from build123d import *

# Parameters (mm, degrees)
ESQUISSE1_W             = 40
ESQUISSE1_H             = 45
ESQUISSE1_R             = 1.75
BOSS_EXTRU_1_DEPTH      = 10
ESQUISSE2_R             = 4
ENL_V_MAT_EXTRU_2_DEPTH = 5
BOSS_EXTRU_2_DEPTH      = 10
ESQUISSE4_W             = 5
ESQUISSE4_H             = 50
BOSS_EXTRU_3_DEPTH      = 20
ENL_V_MAT_EXTRU_3_REACH = 106.163
ESQUISSE5_R             = 3.25
ESQUISSE7_R             = 2.75
BOSS_EXTRU_4_DEPTH      = 10
ENL_V_MAT_EXTRU_5_REACH = 115.719
ESQUISSE8_R             = 15
CHANFREIN1_SIZE         = 15
ENL_V_MAT_EXTRU_4_REACH = 105.475
CHANFREIN3_SIZE         = 3.5


with BuildPart() as part:
    # Esquisse1 → Boss.-Extru.1 (new body)
    with BuildSketch(Plane.XY):
        with Locations((-20, 22.5)):
            Rectangle(ESQUISSE1_W, ESQUISSE1_H)
        with Locations((-16.5, 32.5)):
            Circle(ESQUISSE1_R, mode=Mode.SUBTRACT)
        with Locations((-36.5, 32.5)):
            Circle(ESQUISSE1_R, mode=Mode.SUBTRACT)
        with Locations((-36.5, 12.5)):
            Circle(ESQUISSE1_R, mode=Mode.SUBTRACT)
        with Locations((-16.5, 12.5)):
            Circle(ESQUISSE1_R, mode=Mode.SUBTRACT)
    extrude(amount=BOSS_EXTRU_1_DEPTH)

    # Esquisse2 → Enlèv. mat.-Extru.2 (cut)
    with BuildSketch(Plane.XY.offset(10)):
        with Locations((-36.5, 32.5)):
            Circle(ESQUISSE2_R)
        with Locations((-16.5, 32.5)):
            Circle(ESQUISSE2_R)
        with Locations((-36.5, 12.5)):
            Circle(ESQUISSE2_R)
        with Locations((-16.5, 12.5)):
            Circle(ESQUISSE2_R)
    extrude(amount=-ENL_V_MAT_EXTRU_2_DEPTH, mode=Mode.SUBTRACT)

    # Esquisse3 → Boss.-Extru.2 (add)
    with BuildSketch(Plane.ZY):
        Polygon((10, 0), (45, 35), (45, 85), (40, 85), (0, 45), (10, 45), align=None)
    extrude(amount=BOSS_EXTRU_2_DEPTH)

    # Esquisse4 → Boss.-Extru.3 (add)
    with BuildSketch(Plane.ZY.offset(10)):
        with Locations((42.5, 60)):
            Rectangle(ESQUISSE4_W, ESQUISSE4_H)
    extrude(amount=BOSS_EXTRU_3_DEPTH)

    # Esquisse5 → Enlèv. mat.-Extru.3 (cut, up to next)
    with BuildSketch(Plane.XY.offset(45), mode=Mode.PRIVATE) as enl_v_mat_extru_3_sk1:
        with Locations((-21.5, 70)):
            Circle(ESQUISSE5_R)
    enl_v_mat_extru_3_tool1 = extrude(enl_v_mat_extru_3_sk1.sketch, amount=-ENL_V_MAT_EXTRU_3_REACH, mode=Mode.PRIVATE) & part.part
    # Esquisse5 → Enlèv. mat.-Extru.3 (cut, up to next)
    with BuildSketch(Plane.XY.offset(45), mode=Mode.PRIVATE) as enl_v_mat_extru_3_sk2:
        with Locations((-21.5, 50)):
            Circle(ESQUISSE5_R)
    enl_v_mat_extru_3_tool2 = extrude(enl_v_mat_extru_3_sk2.sketch, amount=-ENL_V_MAT_EXTRU_3_REACH, mode=Mode.PRIVATE) & part.part
    add(enl_v_mat_extru_3_tool1.solids().sort_by_distance((-21.5, 70, 45))[0], mode=Mode.SUBTRACT)
    add(enl_v_mat_extru_3_tool2.solids().sort_by_distance((-21.5, 50, 45))[0], mode=Mode.SUBTRACT)

    # Esquisse7 → Boss.-Extru.4 (add)
    with BuildSketch(Plane.XZ):
        Polygon((0, 0), (0, 10), (-10, 10), (-31.3834406, 29), (-43.3834406, 29), (-43.3834406, 0), align=None)
        with Locations(Location((-37.3834406, 22, 0), (0, 0, 270))):
            Circle(ESQUISSE7_R, mode=Mode.SUBTRACT)
    extrude(amount=BOSS_EXTRU_4_DEPTH)

    # Esquisse8 → Enlèv. mat.-Extru.5 (cut, up to next)
    with BuildSketch(Plane.XZ.offset(10), mode=Mode.PRIVATE) as enl_v_mat_extru_5_sk1:
        with Locations((-56.3834406, 22)):
            Circle(ESQUISSE8_R)
    enl_v_mat_extru_5_tool1 = extrude(enl_v_mat_extru_5_sk1.sketch, amount=-ENL_V_MAT_EXTRU_5_REACH, mode=Mode.PRIVATE) & part.part
    add(enl_v_mat_extru_5_tool1.solids().sort_by_distance((-56.383441, -10, 22))[0], mode=Mode.SUBTRACT)

    # Chanfrein1
    # the kernel refuses this chamfer: 15 mm, written as the material it adds along each edge
    with BuildSketch(Plane(origin=(-10, 35, 40), x_dir=(0, 0, -1), z_dir=(0, 1, 0))) as chanfrein1_piece_1_section:
        Polygon((CHANFREIN1_SIZE, 0), (0, CHANFREIN1_SIZE), (0, 0), align=None)
    chanfrein1_piece_1 = extrude(amount=88.575244819, mode=Mode.PRIVATE)
    chanfrein1_piece_1 = split(chanfrein1_piece_1, bisect_by=Plane(origin=(-10, 60, 15), z_dir=(0, -0.707106781186543, 0.7071067811865521)), keep=Keep.TOP, mode=Mode.PRIVATE)
    chanfrein1_piece_1 = chanfrein1_piece_1 - Plane(origin=(-21.5, 50, 40), x_dir=(1, 0, 0), z_dir=(0, 0, 1)) * Cylinder(3.25, 238, mode=Mode.PRIVATE)
    chanfrein1_piece_1 = chanfrein1_piece_1 - Plane(origin=(-21.5, 70, 40), x_dir=(1, 0, 0), z_dir=(0, 0, 1)) * Cylinder(3.25, 238, mode=Mode.PRIVATE)
    add(chanfrein1_piece_1)
    with BuildSketch(Plane(origin=(-10, 83.575244819, 10), x_dir=(0, 0, 1), z_dir=(0, -1, 0))) as chanfrein1_piece_2_section:
        Polygon((CHANFREIN1_SIZE, 0), (0, CHANFREIN1_SIZE), (0, 0), align=None)
    chanfrein1_piece_2 = extrude(amount=122.150489639, mode=Mode.PRIVATE)
    chanfrein1_piece_2 = split(chanfrein1_piece_2, bisect_by=Plane(origin=(-10, 69.28762241, 24.28762241), z_dir=(0, -0.707106781186543, 0.7071067811865521)), keep=Keep.TOP, mode=Mode.PRIVATE)
    chanfrein1_piece_2 = split(chanfrein1_piece_2, bisect_by=Plane(origin=(-10, 41.78762241, 51.78762241), z_dir=(0, 0.7071067811865328, -0.7071067811865622)), keep=Keep.TOP, mode=Mode.PRIVATE)
    chanfrein1_piece_2 = chanfrein1_piece_2 - Plane(origin=(-16.5, 12.5, 10), x_dir=(1, 0, 0), z_dir=(0, 0, 1)) * Cylinder(4, 305, mode=Mode.PRIVATE)
    chanfrein1_piece_2 = chanfrein1_piece_2 - Plane(origin=(-16.5, 32.5, 10), x_dir=(1, 0, 0), z_dir=(0, 0, 1)) * Cylinder(4, 305, mode=Mode.PRIVATE)
    chanfrein1_piece_2 = split(chanfrein1_piece_2, bisect_by=Plane(origin=(1.78762241, 71.78762241, 10), z_dir=(0.7071067811865477, -0.7071067811865474, 0)), keep=Keep.TOP, mode=Mode.PRIVATE)
    add(chanfrein1_piece_2)
    with BuildSketch(Plane(origin=(-10, 83.575244819, 10), x_dir=(0, 0, 1), z_dir=(0, -1, 0))) as chanfrein1_piece_3_section:
        Polygon((CHANFREIN1_SIZE, 0), (0, CHANFREIN1_SIZE), (0, 0), align=None)
    chanfrein1_piece_3 = extrude(amount=83.575244819, mode=Mode.PRIVATE)
    chanfrein1_piece_3 = split(chanfrein1_piece_3, bisect_by=Plane(origin=(-10, 41.78762241, 51.78762241), z_dir=(0, -0.7071067811865328, 0.7071067811865622)), keep=Keep.TOP, mode=Mode.PRIVATE)
    chanfrein1_piece_3 = split(chanfrein1_piece_3, bisect_by=Plane(origin=(-10, 83.575244819, 10), z_dir=(-0.6642173069108601, 0, -0.7475395435694919)), keep=Keep.TOP, mode=Mode.PRIVATE)
    add(chanfrein1_piece_3)
    with BuildSketch(Plane(origin=(-10, 45, -38.575244819), x_dir=(-1, 0, 0), z_dir=(0, 0, 1))) as chanfrein1_piece_4_section:
        Polygon((CHANFREIN1_SIZE, 0), (0, -CHANFREIN1_SIZE), (0, 0), align=None)
    chanfrein1_piece_4 = extrude(amount=87.150489639, mode=Mode.PRIVATE)
    chanfrein1_piece_4 = split(chanfrein1_piece_4, bisect_by=Plane(origin=(-10, 25.71237759, -19.28762241), z_dir=(0, -0.707106781186543, 0.7071067811865521)), keep=Keep.TOP, mode=Mode.PRIVATE)
    chanfrein1_piece_4 = split(chanfrein1_piece_4, bisect_by=Plane(origin=(-41.78762241, 45, -6.78762241), z_dir=(0.7071067811865476, 0, -0.7071067811865476)), keep=Keep.TOP, mode=Mode.PRIVATE)
    add(chanfrein1_piece_4)

    # Esquisse6 → Enlèv. mat.-Extru.4 (cut, up to next)
    with BuildSketch(Plane(origin=(0, 0, 40), x_dir=(-1, 0, 0), z_dir=(0, 0, -1)), mode=Mode.PRIVATE) as enl_v_mat_extru_4_sk1:
        with BuildLine():
            Line((13.5, 70), (13.5, 85))
            Line((13.5, 85), (29.5, 85))
            Line((29.5, 85), (29.5, 70))
            ThreePointArc((29.5, 70), (21.5, 62), (13.5, 70))
        make_face()
    enl_v_mat_extru_4_tool1 = extrude(enl_v_mat_extru_4_sk1.sketch, amount=ENL_V_MAT_EXTRU_4_REACH, mode=Mode.PRIVATE) & part.part
    # Esquisse6 → Enlèv. mat.-Extru.4 (cut, up to next)
    with BuildSketch(Plane(origin=(0, 0, 40), x_dir=(-1, 0, 0), z_dir=(0, 0, -1)), mode=Mode.PRIVATE) as enl_v_mat_extru_4_sk2:
        with BuildLine():
            Line((29.5, 50), (29.5, 35))
            Line((29.5, 35), (13.5, 35))
            Line((13.5, 35), (13.5, 50))
            ThreePointArc((13.5, 50), (21.5, 58), (29.5, 50))
        make_face()
    enl_v_mat_extru_4_tool2 = extrude(enl_v_mat_extru_4_sk2.sketch, amount=ENL_V_MAT_EXTRU_4_REACH, mode=Mode.PRIVATE) & part.part
    add(enl_v_mat_extru_4_tool1.solids().sort_by_distance((-21.5, 74.283507, 40))[0], mode=Mode.SUBTRACT)
    add(enl_v_mat_extru_4_tool2.solids().sort_by_distance((-21.5, 45.716493, 40))[0], mode=Mode.SUBTRACT)

    # Chanfrein3
    # the kernel refuses this chamfer: 3.5 mm, written as the material it adds along each edge
    with BuildSketch(Plane(origin=(-10, 35, 15.999109542), x_dir=(0, -1, 0), z_dir=(0, 0, 1))) as chanfrein3_piece_1_section:
        Polygon((CHANFREIN3_SIZE, 0), (0, -CHANFREIN3_SIZE), (0, 0), align=None)
    chanfrein3_piece_1 = extrude(amount=38.001780916, mode=Mode.PRIVATE)
    chanfrein3_piece_1 = split(chanfrein3_piece_1, bisect_by=Plane(origin=(-10, 20.499554771, 30.499554771), z_dir=(0, 0.7071067811865476, -0.7071067811865476)), keep=Keep.TOP, mode=Mode.PRIVATE)
    chanfrein3_piece_1 = split(chanfrein3_piece_1, bisect_by=Plane(origin=(-5.499554771, 35, 20.499554771), z_dir=(0.7071067811865476, 0, 0.7071067811865476)), keep=Keep.TOP, mode=Mode.PRIVATE)
    add(chanfrein3_piece_1)


solid = part.part
Geometry check sheet. Reference: the model listing, model coordinates, mm. A direction names the side the tool comes from. Give positions to 0.01 mm unless a question says otherwise; leave off trailing zeros. Write each loop counter-clockwise with the first axis right and the second up, starting at its lowest first coordinate (ties: lowest second). Pieces come first, ordered by that corner, then holes. Notation, with made-up numbers: M 39.5,28 L 51.5,28 A30 ccw 51.5,60 Z; hole C 82,57 d10. An arc over 180 degrees is marked long. Answer as CSV lines item,"result". Start each with the question number.
Q1. Section check A-A, the plane y = 32.5. Record the cut outline in (x, z).
Q2. Go/stop test with flat-tipped pins: pin 1 (2 mm diameter, centred on y = 38, z = 21.5, fed in from +X); pin 2 (4 mm diameter, centred on x = -38, y = 11.5, fed in from +Z); pin 3 (8 mm diameter, centred on x = -16.5, y = 52, fed in from -Z); pin 4 (12 mm diameter, centred on x = -33.5, y = 23.5, fed in from +Z). Record where each tip stops, or that it passes through.
Q3. Tool access check on faces 4 (the face through (-10, 25, 31)), 5 (the face through (-15.933, 64.255, 35.608)), 6 (the face through (-12.685, 33.701, 11.928)). Record the directions out of +Z, -Z, +X, -X, +Y, -Y that give a thin tool (end or side, any length) a straight path to the whole face; none if there is none.
Q4. Release check for a two-part mould opening along Y. For faces 1 (the face through (-7, 65, 20)), 2 (the face through (-14.78, 31.67, 5)), 3 (the face through (-20.542, -5.142, 19.367)) record: pulls with the +Y half, pulls with the -Y half, needs draft (parallel to the pull), parting line crosses it, or undercut.
Q5. Material ranges on L1, parallel to Y at x = -36.5, z = 8.45; L2, parallel to Y at x = -16.5, z = 10.5; L3, parallel to Z at x = -1.5, y = -3.5, recorded low to high.
Q6. Section check B-B, the plane x = -9. Record the cut outline in (y, z).
Q7. Section check D-D, the plane z = 8. Record the cut outline in (x, y).
Q8. Section check C-C, the plane y = 68. Record the cut outline in (x, z), then the cut area to 3 significant figures.
Geometry says:
1,outline,"M -40,0 L -38.25,0 L -38.25,5 L -40,5 Z; M -34.75,0 L -18.25,0 L -18.25,5 L -20.5,5 L -20.5,14.5 L -25,10 L -32.5,10 L -32.5,5 L -34.75,5 Z; M -14.75,0 L 0,0 L 0,42.5 L -11,42.5 L -11,26 L -10,25 L -12.5,22.5 L -12.5,5 L -14.75,5 Z"
2,pin 1,"x = 0"
2,pin 2,"z = 5"
2,pin 3,"z = 3"
2,pin 4,"z = 10"
3,face 4,"+Z, -X, -Y"
3,face 5,"-Z, +Y"
3,face 6,"none"
4,face 1,"pulls with the +Y half"
4,face 2,"undercut"
4,face 3,"needs draft"
5,L1,"-10 to 8.5, 16.5 to 28.5, 36.5 to 45"
5,L2,"-10 to 8.5, 16.5 to 28.5, 36.5 to 53.5"
5,L3,"0 to 10"
6,outline,"M -10,0 L 45,0 L 85,40 L 85,45 L 35,45 L 0,10 L -10,10 Z"
7,outline,"M -43.38,-10 L 0,-10 L 0,53 L -17,53 L -25,45 L -40,45 L -40,34.44 A4 cw long -40,30.56 L -40,14.44 A4 cw long -40,10.56 L -40,0 L -43.38,0 Z; hole C -16.5,12.5 d8; hole C -16.5,32.5 d8"
8,outline,"M -30,40 L -24.06,40 L -24.06,45 L -30,45 Z; M -18.94,40 L -13.75,40 L -13.75,28.75 L -10,25 L -10,23 L 0,23 L 0,45 L -18.94,45 Z"
8,area,"344 mm^2"
